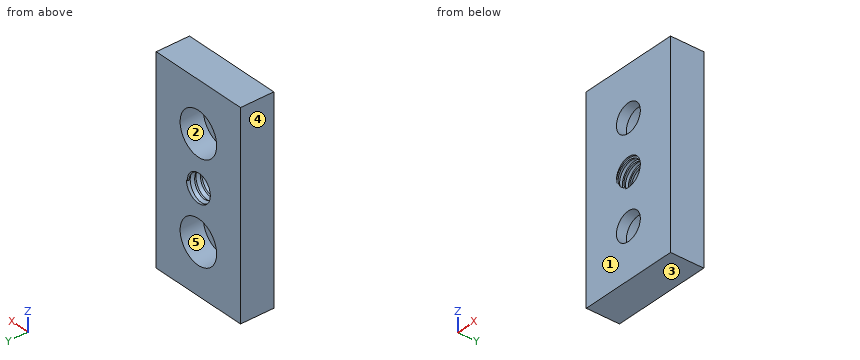
from build123d import *

# Parameters (mm, degrees)
SKETCH_1_W          = 30
SKETCH_1_H          = 60
SKETCH_1_R          = 4.25
EXTRUDE_1_DEPTH     = 10
SKETCH_3_R          = 6.5
CUT_EXTRUDE_1_DEPTH = 7
SWEEP_1_PITCH       = 1.75
SWEEP_1_HEIGHT      = 10
SWEEP_1_RADIUS      = 4.25
SWEEP_1_START_ANGLE = 90
SKETCH_6_W          = 30
SKETCH_6_H          = 9.258755221
SKETCH_6_H_2        = 12.64673583
CUT_EXTRUDE_2_DEPTH = 63.748440843


with BuildPart() as part:
    # 草图1 → 凸台-拉伸1 (new body)
    with BuildSketch(Plane(origin=(0, 0, 0), x_dir=(1, 0, 0), z_dir=(0, 1, 0))):
        Rectangle(SKETCH_1_W, SKETCH_1_H)
        with Locations(Location((0, 15, 0), (0, 0, 270))):
            Circle(SKETCH_1_R, mode=Mode.SUBTRACT)
        with Locations(Location((0, -15, 0), (0, 0, 270))):
            Circle(SKETCH_1_R, mode=Mode.SUBTRACT)
        with Locations(Location((0, 0, 0), (0, 0, 270))):
            Circle(SKETCH_1_R, mode=Mode.SUBTRACT)
    extrude(amount=EXTRUDE_1_DEPTH)

    # 草图3 → 切除-拉伸1 (cut)
    with BuildSketch(Plane(origin=(0, 10, 0), x_dir=(1, 0, 0), z_dir=(0, 1, 0))):
        with Locations(Location((0, 15, 0), (0, 0, 270))):
            Circle(SKETCH_3_R)
        with Locations(Location((0, -15, 0), (0, 0, 270))):
            Circle(SKETCH_3_R)
    extrude(amount=-CUT_EXTRUDE_1_DEPTH, mode=Mode.SUBTRACT)

    # 扫描1: sweep along a helix
    with BuildLine() as sweep_1_path:
        add(Helix(SWEEP_1_PITCH, SWEEP_1_HEIGHT, SWEEP_1_RADIUS, center=(0, 10, 0), direction=(0, -1, 0), mode=Mode.PRIVATE).rotate(Axis((0, 10, 0), (0, -1, 0)), SWEEP_1_START_ANGLE))
    # 草图5 → 扫描1 (sweep)
    with BuildSketch(Plane(origin=(4.25, 10, 0), x_dir=(1, 0, 0), z_dir=(3.1170229136343766e-15, -0.06539411290163802, 0.9978595141590864))):
        Polygon((0, 0.601609008), (-0.521008684, -0.300804504), (0.521008684, -0.300804504), align=None)
    sweep(path=sweep_1_path.line, is_frenet=True)

    # 草图6 → 切除-拉伸2 (cut, through all)
    with BuildSketch(Plane.XY.offset(30)):
        with Locations((0, 14.629377611)):
            Rectangle(SKETCH_6_W, SKETCH_6_H)
        with Locations((0, -6.323367915)):
            Rectangle(SKETCH_6_W, SKETCH_6_H_2)
    extrude(amount=-CUT_EXTRUDE_2_DEPTH, mode=Mode.SUBTRACT)


solid = part.part
Read the model definition and answer for the solid it produces. Units are mm, in the model's axes. Face numbers are marked on the shaded views. A direction names the side the tool comes from. Give positions to 0.01 mm unless a question says otherwise; leave off trailing zeros. Loops run counter-clockwise (first coordinate to the right, second up) from the corner with the lowest first, then second, coordinate; pieces in that order, holes last. Notation, with made-up numbers: (77.25, 69.25) -> (107.25, 69.25) arc R10 ccw to (107.25, 87.25) -> close; hole circle Ø10 at (16, 60.25). An arc over 180 degrees is marked (long way). Use a Markdown table: item, result.
Q1. Determine the mould class of the marked faces 3, 4 and 5 for opening direction Z: pulls with the +Z half, pulls with the -Z half, needs draft (parallel to the pull), parting line crosses it, or undercut.
Solved:
| item | result |
|---|---|
| face 3 | pulls with the -Z half |
| face 4 | needs draft |
| face 5 | undercut |
Q2. Section A-A, the plane z = -15 is taken. Determine the outline of the cut face in (x, y).
Solved:
| item | result |
|---|---|
| outline | (-15, 0) -> (-4.25, 0) -> (-4.25, 3) -> (-6.5, 3) -> (-6.5, 10) -> (-15, 10) -> close; (4.25, 0) -> (15, 0) -> (15, 10) -> (6.5, 10) -> (6.5, 3) -> (4.25, 3) -> close |
Q3. Section B-B, the plane x = 1 is taken. Count the separate pieces of the cut face and the enclosed holes in it, then the cut area to 3 significant figures.
Solved:
| item | result |
|---|---|
| separate pieces | 4 |
| enclosed holes | 0 |
| area | 291 mm^2 |
Q4. A tool of negligible diameter and unlimited length cuts with its end or side. For the marked faces 1 and 2, from which of +Z, -Z, +X, -X, +Y, -Y can it reach the whole face along a straight path? Write none if from no direction.
Solved:
| item | result |
|---|---|
| face 1 | +Z, -Z, +X, -X, -Y |
| face 2 | +Y |
Q5. Find the intervals of material crossed by line 1 along X through (y, z) = (2.45, -15); line 2 along Z through (x, y) = (2.5, 5.75); line 3 along Z through (x, y) = (2, 2.25), in increasing order.
Solved:
| item | result |
|---|---|
| line 1 | x = -15 to -4.25, 4.25 to 15 |
| line 2 | z = -30 to -21, -9 to -3.44, 3.44 to 9, 21 to 30 |
| line 3 | z = -30 to -18.75, -11.25 to -3.75, 3.75 to 11.25, 18.75 to 30 |
Q6. Section C-C, the plane z = 15.5 is taken. Determine the outline of the cut face in (x, y).
Solved:
| item | result |
|---|---|
| outline | (-15, 0) -> (-4.22, 0) -> (-4.22, 3) -> (-6.48, 3) -> (-6.48, 10) -> (-15, 10) -> close; (4.22, 0) -> (15, 0) -> (15, 10) -> (6.48, 10) -> (6.48, 3) -> (4.22, 3) -> close |
Q7. Each of these flat-tipped pins is pushed along its axis until it touches: pin 1 (4 mm diameter, centred on x = -0.5, z = 8, fed in from -Y); pin 2 (7 mm diameter, centred on x = 0, z = 0, fed in from +Y); pin 3 (6.5 mm diameter, centred on x = 2.5, z = 13, fed in from +Y). Where does it stop, or does it pass through?
Solved:
| item | result |
|---|---|
| pin 1 | stops at y = 0 |
| pin 2 | passes through |
| pin 3 | stops at y = 3 |
